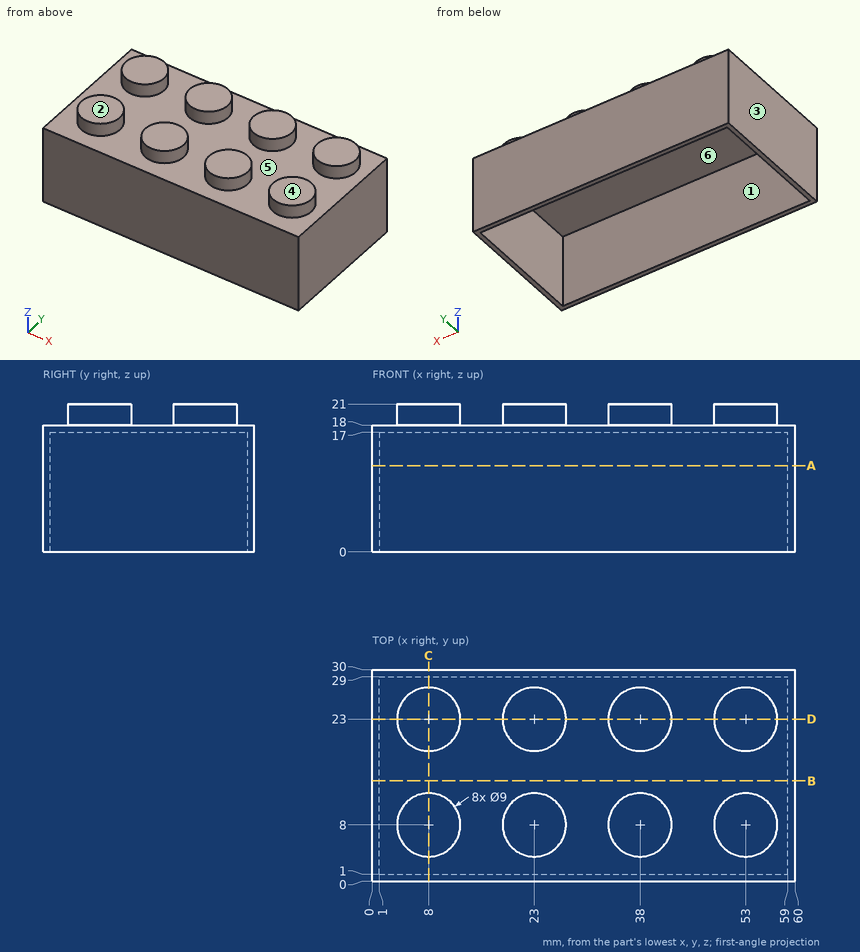
Source: three-view drawing plus pictorial views. Frame: mm from the lowest corner of the part. A direction names the side the tool comes from. Give positions to 0.01 mm unless a question says otherwise; leave off trailing zeros. Write each loop counter-clockwise with the first axis right and the second up, starting at its lowest first coordinate (ties: lowest second). Pieces come first, ordered by that corner, then holes.
(1) Cut plane D-D, the plane y = 23. Return loops of the section in (x, z).
(2) Cut plane B-B, the plane y = 14.25. Return loops of the section in (x, z), then the cut area to 3 significant figures.
(3) Ray query, line 1 (Y direction, x = 27, z = 15.75); line 2 (X direction, y = 21.5, z = 8.5); line 3 (Z direction, x = 22.5, y = 25.25). Return the intervals inside material, ascending.
(4) Cut plane C-C, the plane x = 8. Return loops of the section in (y, z), then the cut area to 3 significant figures.
(5) First-contact query: P1, Ø8.5, axis at x = 30, z = 6.5, coming from the -Y side; P2, Ø1, axis at x = 8.5, y = 17.5, coming from the -Z side; P3, Ø10, axis at x = 15, y = 14.5, coming from the +Z side. Flat tips, straight axial feed; report the tip coordinate or a pass-through.
(6) Access query for the marked faces 4, 5 and 6. Directions: +Z, -Z, +X, -X, +Y, -Y. A direction counts if a zero-diameter tool reaches every point of the face in a straight line with its end or side. Return the directions, or none.
(7) Cut plane A-A, the plane z = 12.25. Return loops of the section in (x, y), then the cut area to 3 significant figures.
(8) Mould query, pull axis X, two halves, no side actions, for the marked faces 1, 2 and 3. Classes: released by +X, released by -X, zero draft, split by the parting line, or undercut.
Values follow:
1. outline: (0, 0) - (1, 0) - (1, 17) - (59, 17) - (59, 0) - (60, 0) - (60, 18) - (57.5, 18) - (57.5, 21) - (48.5, 21) - (48.5, 18) - (42.5, 18) - (42.5, 21) - (33.5, 21) - (33.5, 18) - (27.5, 18) - (27.5, 21) - (18.5, 21) - (18.5, 18) - (12.5, 18) - (12.5, 21) - (3.5, 21) - (3.5, 18) - (0, 18) - close
2. outline: (0, 0) - (1, 0) - (1, 17) - (59, 17) - (59, 0) - (60, 0) - (60, 18) - (0, 18) - close
2. area: 94.0 mm2
3. line 1: y = 0 to 1, 29 to 30
3. line 2: x = 0 to 1, 59 to 60
3. line 3: z = 17 to 21
4. outline: (0, 0) - (1, 0) - (1, 17) - (29, 17) - (29, 0) - (30, 0) - (30, 18) - (27.5, 18) - (27.5, 21) - (18.5, 21) - (18.5, 18) - (12.5, 18) - (12.5, 21) - (3.5, 21) - (3.5, 18) - (0, 18) - close
4. area: 118 mm2
5. P1: stops at y = 0
5. P2: stops at z = 17
5. P3: stops at z = 18
6. face 4: +Z, +X, -X, +Y, -Y
6. face 5: +Z
6. face 6: -Z
7. outline: (0, 0) - (60, 0) - (60, 30) - (0, 30) - close; hole (1, 1) - (59, 1) - (59, 29) - (1, 29) - close
7. area: 176 mm2
8. face 1: undercut
8. face 2: zero draft
8. face 3: released by -X
